The drawing under review shows one solid part. Ordinate dimensions are in mm from its lowest x, y, z. Coordinates: 2 decimals unless noted, no trailing zeros. Order: outer loops, then holes, each group sorted by start corner. A loop starts at its lowest first (then second) coordinate and runs counter-clockwise, first axis right, second up. Notation, with made-up numbers: M 69,-31.75 L 112,-31.75 A15 cw 112,-12.75 Z; hole C 28,87.25 d6. An arc over 180 degrees is marked long. Answer as a JSON object with one key per item and string values.
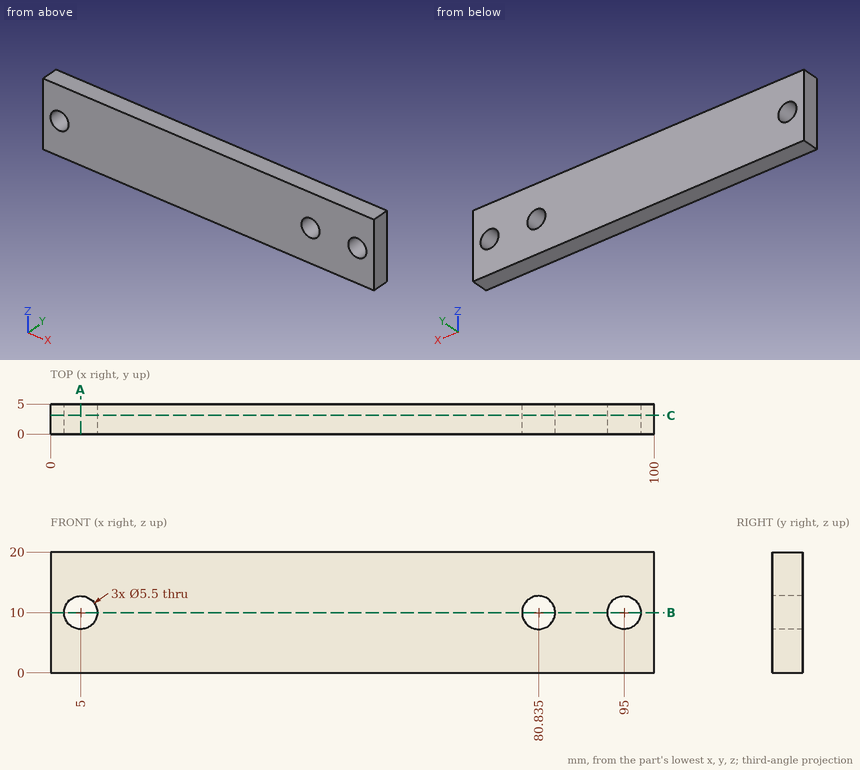
1) Add section A-A (x = 5). State the section outline as (y, z) points, and give its area (3 significant figures).
Taken from the geometry:
{"outline": "M 0,0 L 5,0 L 5,7.25 L 0,7.25 Z; M 0,12.75 L 5,12.75 L 5,20 L 0,20 Z", "area": "72.5 mm2"}
2) Add section C-C (y = 3.1). State the section outline as (x, z) points (3 decimals), and give its area (3 significant figures).
Taken from the geometry:
{"outline": "M 0,0 L 100,0 L 100,20 L 0,20 Z; hole C 5,10 d5.5; hole C 80.835,10 d5.5; hole C 95,10 d5.5", "area": "1,930 mm2"}
3) Insertion check: pin 1 Ø9 at (x, z) = (80.835, 10) entering from -Y; pin 2 Ø4.5 at (x, z) = (95, 10) entering from +Y. Each pin has a flat end and moves straight along its axis. Give the tip position at first contact, or say it passes through.
Taken from the geometry:
{"pin 1": "stops at y = 0", "pin 2": "passes through"}
4) To check wall thickness, follow L1, parallel to Z at x = 95, y = 3.55; L2, parallel to X at y = 0.65, z = 8.5; L3, parallel to Z at x = 96, y = 4.3. State the ranges of each line that lie inside material, in increasing order.
Taken from the geometry:
{"L1": "z = 0 to 7.25, 12.75 to 20", "L2": "x = 0 to 2.7, 7.3 to 78.53, 83.14 to 92.7, 97.3 to 100", "L3": "z = 0 to 7.44, 12.56 to 20"}
5) Add section B-B (z = 10). State the section outline as (x, y) points (3 decimals), and give its area (4 significant figures).
Taken from the geometry:
{"outline": "M 0,0 L 2.25,0 L 2.25,5 L 0,5 Z; M 7.75,0 L 78.085,0 L 78.085,5 L 7.75,5 Z; M 83.585,0 L 92.25,0 L 92.25,5 L 83.585,5 Z; M 97.75,0 L 100,0 L 100,5 L 97.75,5 Z", "area": "417.5 mm2"}
